Print and shaded views of the part. All mm, measured from the part's lowest x, y and z. Coordinates: 2 decimals unless noted, no trailing zeros. Order: outer loops, then holes, each group sorted by start corner. A loop starts at its lowest first (then second) coordinate and runs counter-clockwise, first axis right, second up. Notation, with made-up numbers: M 57.25,16.25 L 75.25,16.25 A16 cw 75.25,40.25 Z; hole C 72,36 d9. An arc over 180 degrees is marked long. Return JSON: item names as keys, results as strings.
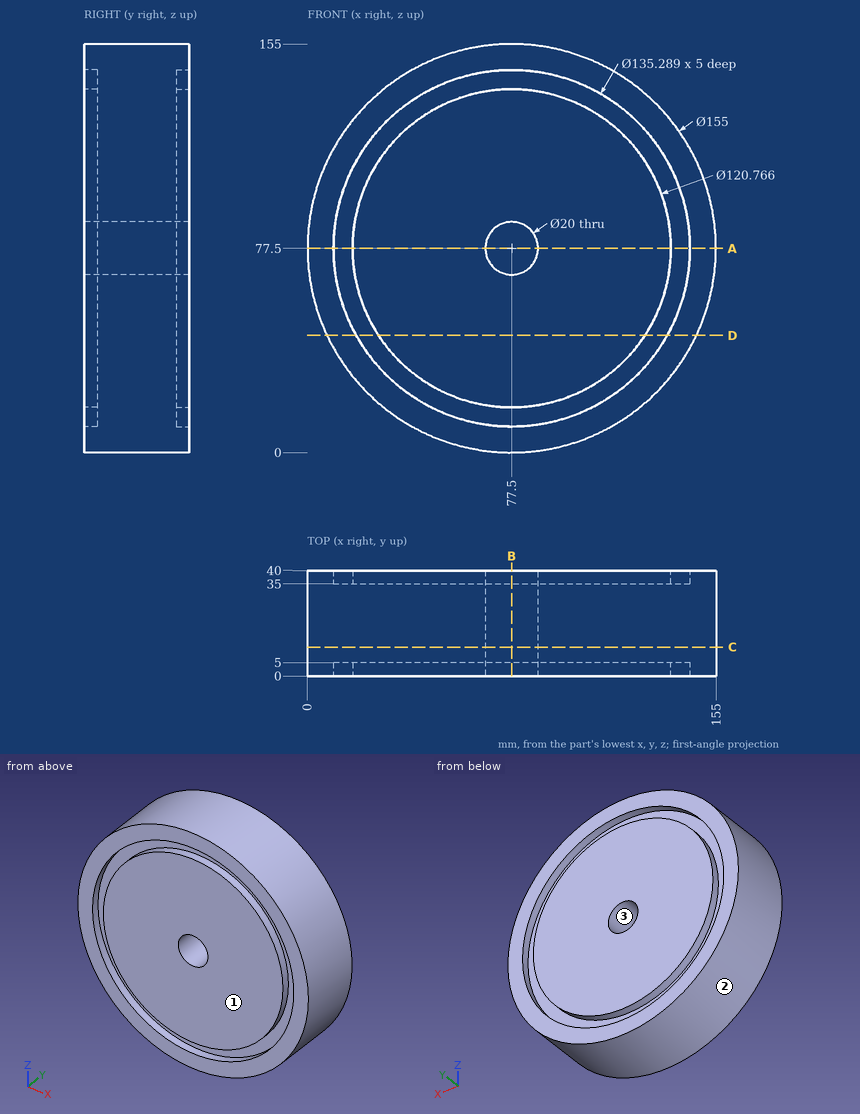
Item 1: Wall check: line 1 (Z direction, x = 77, y = 37); line 2 (Y direction, x = 123.5, z = 38). Give the ranges that are in metal, low to high.
Check result:
{"line 1": "z = 0 to 9.86, 17.12 to 67.51, 87.49 to 137.88, 145.14 to 155", "line 2": "y = 5 to 35"}
Item 2: Drop flat-ended pins along their axis: pin 1 Ø12 at (x, z) = (103.5, 137.5) entering from -Y; pin 2 Ø8 at (y, z) = (33.5, 45.5) entering from +X (1 decimal); pin 3 Ø12 at (y, z) = (18.5, 101.5) entering from -X; pin 4 Ø12 at (x, z) = (77.5, 77.5) entering from -Y. Give the stop position or say it passes through.
Check result:
{"pin 1": "stops at y = 0", "pin 2": "stops at x = 149.8", "pin 3": "stops at x = 2.12", "pin 4": "passes through"}
Item 3: Saw through at A-A (z = 77.5). Write the cut outline in (x, y) (1 decimal).
Check result:
{"outline": "M 0,0 L 9.9,0 L 9.9,5 L 17.1,5 L 17.1,0 L 67.5,0 L 67.5,40 L 17.1,40 L 17.1,35 L 9.9,35 L 9.9,40 L 0,40 Z; M 87.5,0 L 137.9,0 L 137.9,5 L 145.1,5 L 145.1,0 L 155,0 L 155,40 L 145.1,40 L 145.1,35 L 137.9,35 L 137.9,40 L 87.5,40 Z"}
Item 4: Saw through at B-B (x = 77.5). Write the cut outline in (y, z) (1 decimal).
Check result:
{"outline": "M 0,0 L 40,0 L 40,9.9 L 35,9.9 L 35,17.1 L 40,17.1 L 40,67.5 L 0,67.5 L 0,17.1 L 5,17.1 L 5,9.9 L 0,9.9 Z; M 0,87.5 L 40,87.5 L 40,137.9 L 35,137.9 L 35,145.1 L 40,145.1 L 40,155 L 0,155 L 0,145.1 L 5,145.1 L 5,137.9 L 0,137.9 Z"}
Item 5: Saw through at C-C (y = 11). Write the cut outline in (x, z).
Check result:
{"outline": "C 77.5,77.5 d155; hole C 77.5,77.5 d20"}
Item 6: Saw through at D-D (z = 44.5). Write the cut outline in (x, y).
Check result:
{"outline": "M 7.38,0 L 18.45,0 L 18.45,5 L 26.93,5 L 26.93,0 L 128.07,0 L 128.07,5 L 136.55,5 L 136.55,0 L 147.62,0 L 147.62,40 L 136.55,40 L 136.55,35 L 128.07,35 L 128.07,40 L 26.93,40 L 26.93,35 L 18.45,35 L 18.45,40 L 7.38,40 Z"}
Item 7: Pull direction Z, two halves, no side cores. Call the marked faces 1, 2 and 3: +Z half, -Z half, draft (parallel to the pull), parting line (faces both ways), or undercut.
Check result:
{"face 1": "draft", "face 2": "parting line", "face 3": "undercut"}
